The figure shows three views and two pictorial views of one solid part (mm, origin at its lowest corner). Answer the questions. Give positions to 0.01 mm unless a question says otherwise; leave off trailing zeros. Order: outer loops, then holes, each group sorted by start corner. A loop starts at its lowest first (then second) coordinate and runs counter-clockwise, first axis right, second up. Notation, with made-up numbers: M 69.5,-34.75 L 97.5,-34.75 A19 cw 97.5,-4.75 Z; hole C -22,-35 d1. An arc over 180 degrees is marked long. Write item = value, one per line. Start each with the question number.
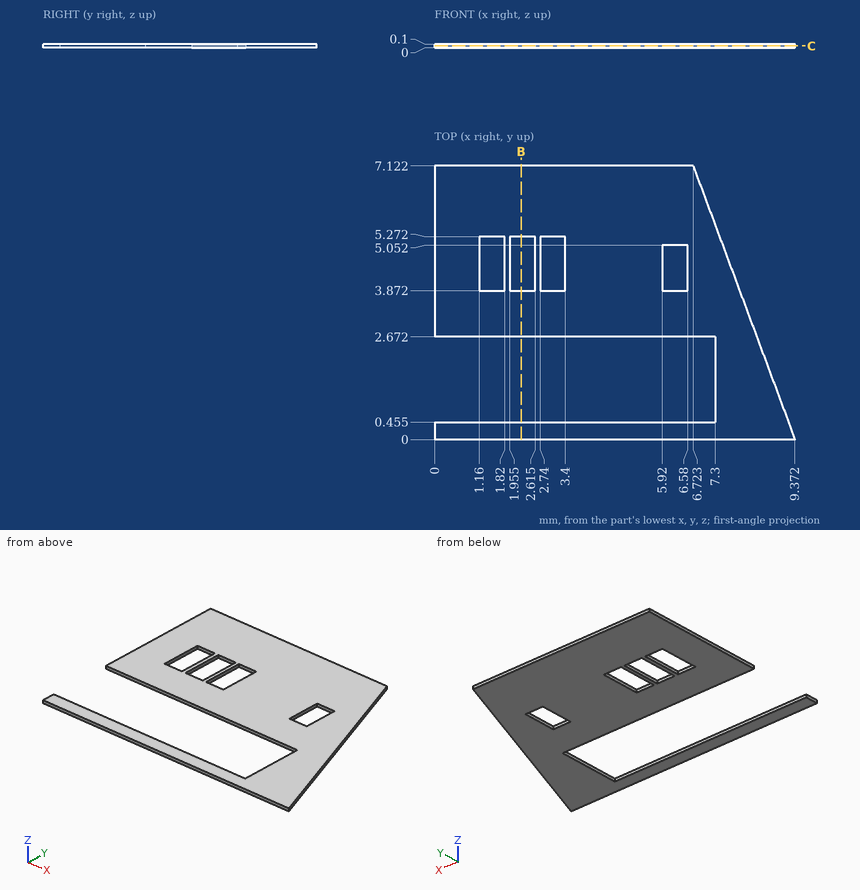
1) Find section B-B on x = 2.25. Count the separate pieces of the cut face and the enclosed holes in it.
2) Find section C-C on z = 0.05. Determine the outline of the cut face in (x, y) (1 decimal).
3) Find the intervals of material crossed by probe 1 along Y at (x, z) = (5.5, 0.05) (1 decimal); probe 2 along X at (y, z) = (3.25, 0.05), in increasing order. Write a range as [from, to].
Numbers:
q1.separate_pieces = 3
q1.enclosed_holes = 0
q2.outline = M 0,0 L 9.4,0 L 6.7,7.1 L 0,7.1 L 0,2.7 L 7.3,2.7 L 7.3,0.5 L 0,0.5 Z; hole M 1.2,3.9 L 1.8,3.9 L 1.8,5.3 L 1.2,5.3 Z; hole M 2,3.9 L 2.6,3.9 L 2.6,5.3 L 2,5.3 Z; hole M 2.7,3.9 L 3.4,3.9 L 3.4,5.3 L 2.7,5.3 Z; hole M 5.9,3.9 L 6.6,3.9 L 6.6,5.1 L 5.9,5.1 Z
q3.probe_1 = [0, 0.5], [2.7, 7.1]
q3.probe_2 = [0, 8.16]
